Build history of the part. All positions in model axes, mm. Face numbers are marked on the shaded views. A direction names the side the tool comes from. Give positions to 0.01 mm unless a question says otherwise; leave off trailing zeros. Order: outer loops, then holes, each group sorted by start corner. A loop starts at its lowest first (then second) coordinate and runs counter-clockwise, first axis right, second up. Notation, with made-up numbers: M -22.5,-19 L -9.5,-19 A27 cw -9.5,15 Z; hole C 83,72 d5. An arc over 180 degrees is marked long. Use CSV: the item, a comma, the result in double quotes. Start each with the question number.
Item 1: Band-saw the part on C-C on x = -19. Write the cut outline in (y, z).
Item 2: Which spindle directions (+Z, -Z, +X, -X, +Y, -Y) get a long thin tool onto all of the face, cutting with end or side? Do the marked faces 1 and 2. Say none if no direction does.
Item 3: Pin check, flat tips, straight feed: P1, Ø10, axis at y = -10, z = -12.5, coming from the -X side; P2, Ø1, axis at y = -16, z = 22.5, coming from the +X side; P3, Ø1.8, axis at x = -37, z = 29.5, coming from the -Y side. Stop position of each tip, or through.
Item 4: Wall check: line 1 along X through (y, z) = (-6.75, 27); line 2 along X through (y, z) = (-9.25, 29.5); line 3 along X through (y, z) = (0.25, -29.5). Give the ranges that are in metal, low to high.
Item 5: Band-saw the part on A-A on z = 29.5. Write the cut outline in (x, y), plus the area to 3 significant figures.
Item 6: Two-plate mould, pull along X, no slides. Class the marked faces 3, 4 and 5: pulls with the +X half, pulls with the -X half, needs draft (parallel to the pull), parting line crosses it, or undercut.
Item 7: Band-saw the part on B-B on y = -11.5. Give the number of separate pieces and of enclosed holes in the cut face, plus the area to 3 significant figures.
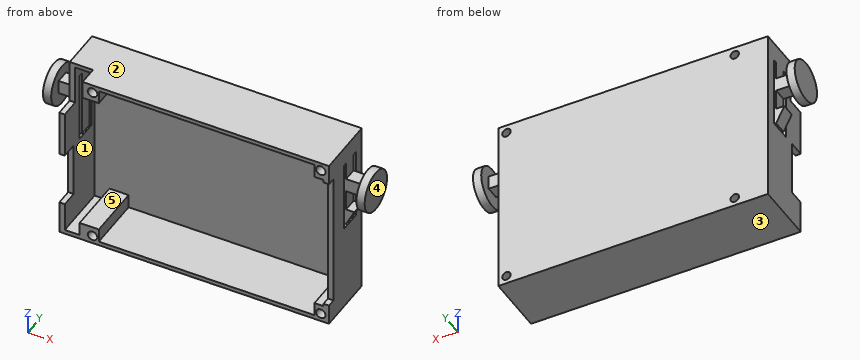
from build123d import *

# Parameters (mm, degrees)
SKETCH_1_W          = 98.5
SKETCH_1_H          = 65
EXTRUDE_1_DEPTH     = 2
SKETCH_2_W          = 98.5
SKETCH_2_H          = 65
SKETCH_2_W_2        = 94.5
SKETCH_2_H_2        = 62
EXTRUDE_2_DEPTH     = 20
SKETCH_3_W          = 20
SKETCH_3_H          = 6
SKETCH_3_W_2        = 15.9
SKETCH_3_H_2        = 7
CUT_EXTRUDE_1_DEPTH = 8.5
CUT_EXTRUDE_5_DEPTH = 106.633801408
SKETCH_8_W          = 6.5
SKETCH_8_H          = 5
EXTRUDE_5_DEPTH     = 5
SKETCH_9_R          = 1.55
CUT_EXTRUDE_7_DEPTH = 69.178534012
SKETCH_10_R         = 2.25
SKETCH_10_R_2       = 1.55
EXTRUDE_6_DEPTH     = 20
SKETCH_11_W         = 50
SKETCH_11_H         = 6
CUT_EXTRUDE_8_DEPTH = 10
EXTRUDE_8_DEPTH     = 20
SKETCH_16_R         = 1.75
CUT_EXTRUDE_9_DEPTH = 15
SKETCH_17_R         = 7.5
EXTRUDE_9_DEPTH     = 3
EXTRUDE_START       = 3
SKETCH_18_R         = 7.5
EXTRUDE_10_DEPTH    = 3


with BuildPart() as part:
    # 草图1 → 凸台-拉伸1 (new body)
    with BuildSketch(Plane(origin=(0, 0, 0), x_dir=(1, 0, 0), z_dir=(0, 1, 0))):
        Rectangle(SKETCH_1_W, SKETCH_1_H)
    extrude(amount=EXTRUDE_1_DEPTH)

    # 草图2 → 凸台-拉伸2 (add)
    with BuildSketch(Plane(origin=(0, 0, 0), x_dir=(-1, 0, 0), z_dir=(0, -1, 0))):
        Rectangle(SKETCH_2_W, SKETCH_2_H)
        Rectangle(SKETCH_2_W_2, SKETCH_2_H_2, mode=Mode.SUBTRACT)
    extrude(amount=EXTRUDE_2_DEPTH)

    # 草图3 → 切除-拉伸1 (cut)
    with BuildSketch(Plane.ZY.offset(49.25)):
        with Locations((-10.4, -17)):
            Rectangle(SKETCH_3_W, SKETCH_3_H)
        with Locations((24.55, -16.5)):
            Rectangle(SKETCH_3_W_2, SKETCH_3_H_2)
    extrude(amount=-CUT_EXTRUDE_1_DEPTH, mode=Mode.SUBTRACT)

    # 草图7 → 切除-拉伸5 (cut, through all)
    with BuildSketch(Plane.ZY.offset(49.25)):
        Polygon((25.5, -3.5), (25.5, -2), (-0.5, -2), (-0.5, -10), (25.5, -10), (25.5, -8.5), (0.5, -8.5), (0.5, -3.5), align=None)
    extrude(amount=-CUT_EXTRUDE_5_DEPTH, mode=Mode.SUBTRACT)

    # 草图8 → 凸台-拉伸5 (add)
    with BuildSketch(Plane(origin=(0, -3.5, 0), x_dir=(1, 0, 0), z_dir=(0, 1, 0))):
        Polygon((-49.25, -0.5), (-52.25, -6.5), (-49.25, -6.5), align=None)
        Polygon((49.25, -0.5), (52.25, -6.5), (49.25, -6.5), align=None)
        with Locations((52.5, -16.5)):
            Rectangle(SKETCH_8_W, SKETCH_8_H)
        with Locations((-52.5, -16.5)):
            Rectangle(SKETCH_8_W, SKETCH_8_H)
    extrude(amount=-EXTRUDE_5_DEPTH)

    # 草图9 → 切除-拉伸7 (cut, through all)
    with BuildSketch(Plane(origin=(0, 2, 0), x_dir=(1, 0, 0), z_dir=(0, 1, 0))):
        with Locations(Location((46.25, 29.5, 0), (0, 0, 270))):
            Circle(SKETCH_9_R)
        with Locations(Location((46.25, -29.5, 0), (0, 0, 270))):
            Circle(SKETCH_9_R)
        with Locations(Location((-37.117, 29.5, 0), (0, 0, 270))):
            Circle(SKETCH_9_R)
        with Locations(Location((-37.117, -29.5, 0), (0, 0, 270))):
            Circle(SKETCH_9_R)
    extrude(amount=-CUT_EXTRUDE_7_DEPTH, mode=Mode.SUBTRACT)

    # 草图10 → 凸台-拉伸6 (add, through all)
    # profile 1 of 4: a face of its own
    with BuildSketch(Plane(origin=(0, 0, 0), x_dir=(-1, 0, 0), z_dir=(0, -1, 0))):
        with Locations((-46.25, 29.5)):
            Circle(SKETCH_10_R)
        with Locations(Location((-46.25, 29.5, 0), (0, 0, 270))):
            Circle(SKETCH_10_R_2, mode=Mode.SUBTRACT)
    # profile 2 of 4: a face of its own
    with BuildSketch(Plane(origin=(0, 0, 0), x_dir=(-1, 0, 0), z_dir=(0, -1, 0))):
        with Locations((37.117, 29.5)):
            Circle(SKETCH_10_R)
        with Locations(Location((37.117, 29.5, 0), (0, 0, 270))):
            Circle(SKETCH_10_R_2, mode=Mode.SUBTRACT)
    # profile 3 of 4: a face of its own
    with BuildSketch(Plane(origin=(0, 0, 0), x_dir=(-1, 0, 0), z_dir=(0, -1, 0))):
        with Locations((-46.25, -29.5)):
            Circle(SKETCH_10_R)
        with Locations(Location((-46.25, -29.5, 0), (0, 0, 270))):
            Circle(SKETCH_10_R_2, mode=Mode.SUBTRACT)
    # profile 4 of 4: a face of its own
    with BuildSketch(Plane(origin=(0, 0, 0), x_dir=(-1, 0, 0), z_dir=(0, -1, 0))):
        with Locations((37.117, -29.5)):
            Circle(SKETCH_10_R)
        with Locations(Location((37.117, -29.5, 0), (0, 0, 270))):
            Circle(SKETCH_10_R_2, mode=Mode.SUBTRACT)
    extrude(amount=EXTRUDE_6_DEPTH)

    # 草图11 → 切除-拉伸8 (cut)
    with BuildSketch(Plane(origin=(49.25, 0, 0), x_dir=(0, 0, -1), z_dir=(1, 0, 0))):
        with Locations((0, -20)):
            Rectangle(SKETCH_11_W, SKETCH_11_H)
    extrude(amount=-CUT_EXTRUDE_8_DEPTH, mode=Mode.SUBTRACT)

    # 草图15 → 凸台-拉伸8 (add, through all)
    with BuildSketch(Plane(origin=(0, 0, 0), x_dir=(-1, 0, 0), z_dir=(0, -1, 0))):
        with BuildLine():
            Line((-43.95, 26), (-43.95, 31))
            Line((-43.95, 31), (-44.572949017, 31))
            ThreePointArc((-44.572949017, 31), (-44.459916807, 28.136877788), (-47.25, 27.484435563))
            Line((-47.25, 27.484435563), (-47.25, 26))
            Line((-47.25, 26), (-43.95, 26))
        make_face()
        with BuildLine():
            Line((-44.572949017, -31), (-43.95, -31))
            Line((-43.95, -31), (-43.95, -26))
            Line((-43.95, -26), (-47.25, -26))
            Line((-47.25, -26), (-47.25, -27.484435563))
            ThreePointArc((-47.25, -27.484435563), (-44.459916807, -28.136877788), (-44.572949017, -31))
        make_face()
        with BuildLine():
            Line((35.439949017, 31), (34.817, 31))
            Line((34.817, 31), (34.817, 26))
            Line((34.817, 26), (41.817, 26))
            Line((41.817, 26), (41.817, 31))
            Line((41.817, 31), (38.794050983, 31))
            ThreePointArc((38.794050983, 31), (37.117, 27.25), (35.439949017, 31))
        make_face()
        with BuildLine():
            Line((34.817, -26), (34.817, -31))
            Line((34.817, -31), (35.439949017, -31))
            ThreePointArc((35.439949017, -31), (37.117, -27.25), (38.794050983, -31))
            Line((38.794050983, -31), (40.75, -31))
            Line((40.75, -31), (40.75, -26))
            Line((40.75, -26), (34.817, -26))
        make_face()
    extrude(amount=EXTRUDE_8_DEPTH)

    # 草图16 → 切除-拉伸9 (cut)
    with BuildSketch(Plane(origin=(0, -20, 0), x_dir=(-1, 0, 0), z_dir=(0, -1, 0))):
        with Locations(Location((-46.25, 29.5, 0), (0, 0, 90))):
            Circle(SKETCH_16_R)
        with Locations(Location((37.117, 29.5, 0), (0, 0, 90))):
            Circle(SKETCH_16_R)
        with Locations(Location((37.117, -29.5, 0), (0, 0, 90))):
            Circle(SKETCH_16_R)
        with Locations(Location((-46.25, -29.5, 0), (0, 0, 90))):
            Circle(SKETCH_16_R)
    extrude(amount=-CUT_EXTRUDE_9_DEPTH, mode=Mode.SUBTRACT)

    # 草图17 → 凸台-拉伸9 (add)
    with BuildSketch(Plane(origin=(55.75, 0, 0), x_dir=(0, 0, -1), z_dir=(1, 0, 0))):
        with Locations(Location((-16, -6, 0), (0, 0, 90))):
            Circle(SKETCH_17_R)
    extrude(amount=EXTRUDE_9_DEPTH)

    # 草图18 → 凸台-拉伸10 (add)
    with BuildSketch(Plane.ZY.offset(55.75).offset(EXTRUDE_START)):
        with Locations(Location((16, -6, 0), (0, 0, 90))):
            Circle(SKETCH_18_R)
    extrude(amount=-EXTRUDE_10_DEPTH)


solid = part.part
Model answer:
1,outline,"M -20,-32.5 L 2,-32.5 L 2,32.5 L -20,32.5 L -20,31 L 0,31 L 0,-31 L -20,-31 Z"
2,face 1,"-Y"
2,face 2,"+Z, +X, -X, +Y, -Y"
3,P1,"stops at x = -49.25"
3,P2,"stops at x = 49.25"
3,P3,"passes through"
4,line 1,"x = -49.25 to -47.25, -40.75 to -34.82, 43.95 to 49.25"
4,line 2,"x = -49.25 to -47.25, -40.75 to -38.87, -35.37 to -34.82, 43.95 to 44.5, 48 to 49.25"
4,line 3,"x = -49.25 to -38.67, -35.57 to 44.7, 47.8 to 49.25"
5,outline,"M -49.25,-13 L -47.25,-13 L -47.25,0 L -40.75,0 L -40.75,-20 L -38.87,-20 L -38.87,-5 L -38.67,-5 L -38.67,2 L -49.25,2 Z; M -35.57,-5 L -35.37,-5 L -35.37,-20 L -34.82,-20 L -34.82,0 L 43.95,0 L 43.95,-20 L 44.5,-20 L 44.5,-5 L 44.7,-5 L 44.7,2 L -35.57,2 Z; M 47.8,-5 L 48,-5 L 48,-20 L 49.25,-20 L 49.25,2 L 47.8,2 Z"
5,area,"299 mm^2"
6,face 3,"needs draft"
6,face 4,"pulls with the +X half"
6,face 5,"undercut"
7,separate pieces,"3"
7,enclosed holes,"5"
7,area,"664 mm^2"
